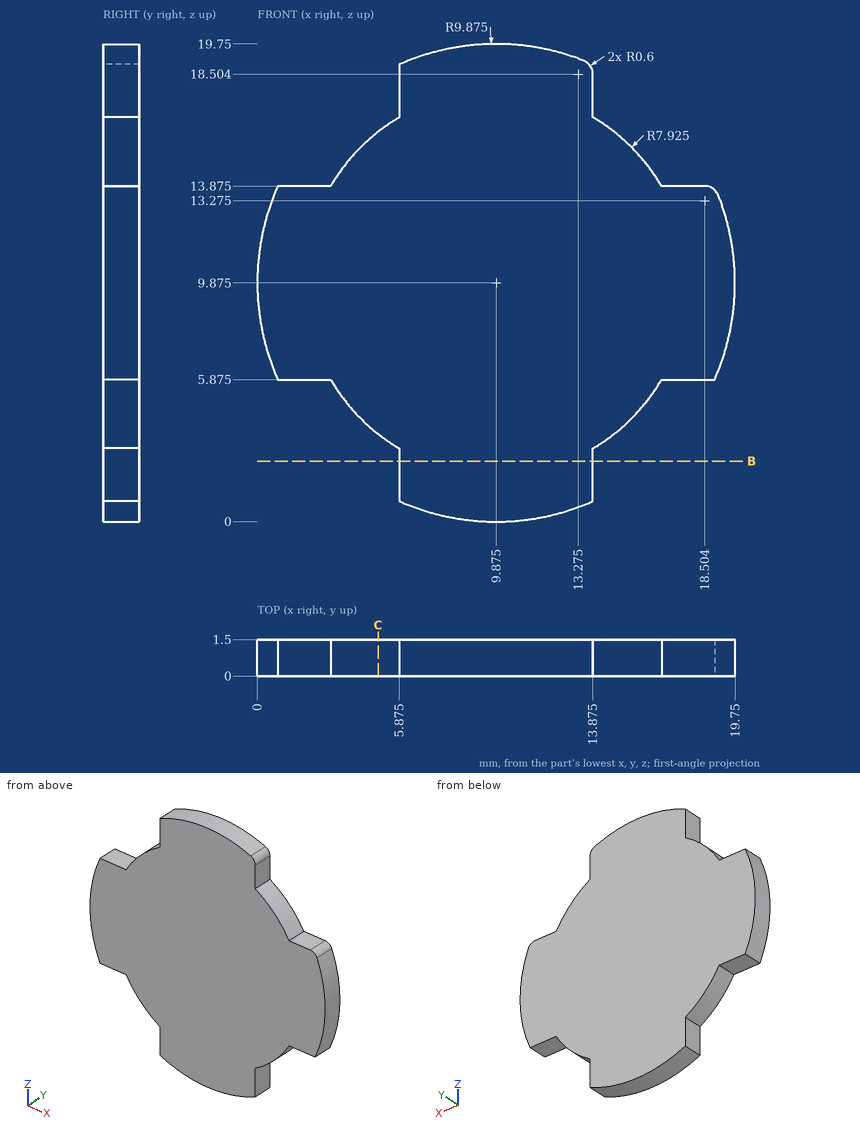
Study the drawing (mm; zero at the part's minimum x, y, z) and answer. Round coordinates to 2 decimals unless told otherwise and drop trailing zeros. Write each loop counter-clockwise with the first axis right and the second up, starting at its lowest first coordinate (ties: lowest second). Pieces come first, ordered by that corner, then holes.
1) A cutting plane is placed at B-B on z = 2.5. Determine the outline of the cut face in (x, y) (1 decimal), and give its area (3 significant figures).
2) Flat-ended cylindrical pins translate along their axes: P1, Ø0.8, axis at x = 17.5, y = 1, coming from the +Z side (3 decimals); P2, Ø0.8, axis at y = 0.5, z = 18, coming from the -X side (3 decimals). Find the tip coordinate at first contact, or state that the pin passes through.
3) Consider probe 1 along Z at (x, y) = (18.5, 0.9) (1 decimal); probe 2 along Z at (x, y) = (11, 0.85) (1 decimal). Determine where each line is inside the solid, lowest interval first.
4) A cutting plane is placed at C-C on x = 5. Determine the outline of the cut face in (y, z).
Entries:
1. outline: (5.9, 0) - (13.9, 0) - (13.9, 1.5) - (5.9, 1.5) - close
1. area: 12.0 mm2
2. P1: stops at z = 13.875
2. P2: stops at x = 5.875
3. probe 1: z = 5.9 to 13.9
3. probe 2: z = 0.1 to 19.7
4. outline: (0, 3.63) - (1.5, 3.63) - (1.5, 16.12) - (0, 16.12) - close
